CAD build for the part. Positions are in the model's coordinates, mm. A direction names the side the tool comes from. Give positions to 0.01 mm unless a question says otherwise; leave off trailing zeros. Write each loop counter-clockwise with the first axis right and the second up, starting at its lowest first coordinate (ties: lowest second). Pieces come first, ordered by that corner, then holes. Notation, with made-up numbers: (-34, -38.5) - (-16, -38.5) arc R21 ccw to (-16, -13.5) - close; hole circle Ø8 at (35, 54). An arc over 180 degrees is marked (long way). Answer as a JSON object with one key per item and string values.
from build123d import *

# Parameters (mm, degrees)
F0_R      = 13.1
F1_DEPTH  = 80
F2_R      = 9.5
F3_DEPTH  = 50
F4_R      = 6.6526235809
F5_DEPTH  = 25
F7_DEPTH  = 25
F8_R      = 0.75
F9_DEPTH  = 5
F10_W     = 4.01619326
F10_H     = 1.2
F11_DEPTH = 1
F13_DEPTH = 44
F14_DEPTH = 44
F15_DEPTH = 10
F16_DEPTH = 10


with BuildPart() as f1:
    # F0 (on Top) → F1 (new body)
    with BuildSketch(Plane.XY):
        Circle(F0_R)
    extrude(amount=F1_DEPTH)

    # F2 (on face) → F3 (cut)
    with BuildSketch(Plane.XY.offset(80)):
        Circle(F2_R)
    extrude(amount=-F3_DEPTH, mode=Mode.SUBTRACT)

    # F4 (on face) → F5 (cut)
    with BuildSketch(Plane.XY.offset(30)):
        Circle(F4_R)
    extrude(amount=-F5_DEPTH, mode=Mode.SUBTRACT)

    # F6 (on face) → F7 (join)
    with BuildSketch(Plane.XY.offset(5)):
        with BuildLine():
            ThreePointArc((2.00809663, 6.3423141229), (0, 6.6526235809), (-2.00809663, 6.3423141229))
            Line((-2.00809663, 6.3423141229), (-2.00809663, -6.3423141229))
            ThreePointArc((-2.00809663, -6.3423141229), (0, -6.6526235809), (2.00809663, -6.3423141229))
            Line((2.00809663, -6.3423141229), (2.00809663, 6.3423141229))
        make_face()
    extrude(amount=F7_DEPTH)

    # F8 (on face) → F9 (cut)
    with BuildSketch(Plane.XY.offset(5)):
        with Locations((-3.75, 0)):
            Circle(F8_R)
        with Locations((3.75, 0)):
            Circle(F8_R)
    extrude(amount=-F9_DEPTH, mode=Mode.SUBTRACT)

    # F10 (on face) → F11 (cut)
    with BuildSketch(Plane.XY.offset(30)):
        Rectangle(F10_W, F10_H)
    extrude(amount=-F11_DEPTH, mode=Mode.SUBTRACT)

    # F12 (on face) → F13 (cut)
    with BuildSketch(Plane.XY.offset(80)):
        with BuildLine():
            Line((-7.3388648552, 10.8513161708), (-4.4335485277, 8.4020025859))
            ThreePointArc((-4.4335485277, 8.4020025859), (1.034452264, 9.4435114504), (6.1473147231, 7.2429635989))
            Line((6.1473147231, 7.2429635989), (7.3388648552, 10.8513161708))
            ThreePointArc((7.3388648552, 10.8513161708), (0, 13.1), (-7.3388648552, 10.8513161708))
        make_face()
    extrude(amount=-F13_DEPTH, mode=Mode.SUBTRACT)

    # F12 (on face) → F14 (cut)
    with BuildSketch(Plane.XY.offset(80)):
        with BuildLine():
            ThreePointArc((4.4335485277, -8.4020025859), (-1.034452264, -9.4435114504), (-6.1473147231, -7.2429635989))
            Line((-6.1473147231, -7.2429635989), (-7.3388648552, -10.8513161708))
            ThreePointArc((-7.3388648552, -10.8513161708), (0, -13.1), (7.3388648552, -10.8513161708))
            Line((7.3388648552, -10.8513161708), (4.4335485277, -8.4020025859))
        make_face()
    extrude(amount=-F14_DEPTH, mode=Mode.SUBTRACT)

    # F12 (on face) → F15 (join)
    with BuildSketch(Plane.XY.offset(80)):
        with BuildLine():
            ThreePointArc((4.4335485277, -8.4020025859), (-1.034452264, -9.4435114504), (-6.1473147231, -7.2429635989))
            Line((-6.1473147231, -7.2429635989), (-7.3388648552, -10.8513161708))
            ThreePointArc((-7.3388648552, -10.8513161708), (0, -13.1), (7.3388648552, -10.8513161708))
            Line((7.3388648552, -10.8513161708), (4.4335485277, -8.4020025859))
        make_face()
    extrude(amount=-F15_DEPTH)

    # F12 (on face) → F16 (join)
    with BuildSketch(Plane.XY.offset(80)):
        with BuildLine():
            Line((-7.3388648552, 10.8513161708), (-4.4335485277, 8.4020025859))
            ThreePointArc((-4.4335485277, 8.4020025859), (1.034452264, 9.4435114504), (6.1473147231, 7.2429635989))
            Line((6.1473147231, 7.2429635989), (7.3388648552, 10.8513161708))
            ThreePointArc((7.3388648552, 10.8513161708), (0, 13.1), (-7.3388648552, 10.8513161708))
        make_face()
    extrude(amount=-F16_DEPTH)


solid = f1.part
(1) Probe L1, parallel to Z at x = -1, y = -9.75; L2, parallel to X at y = 1.5, z = 22; L3, parallel to X at y = 0, z = 53. List the from-to ranges inside material, lowest first. Write a range as [from, to].
Answer key:
{"L1": "z = [0, 36], [70, 80]", "L2": "x = [-13.01, -6.48], [-2.01, 2.01], [6.48, 13.01]", "L3": "x = [-13.1, -9.5], [9.5, 13.1]"}
(2) Pull direction Y, two halves, no side cores. Call faces 5 (the face through (3, 0, 3)), 6 (the face through (9, 4, 80)), 7 (the face through (-6.735, -9.022, 53.238)): pulls with the +Y half, pulls with the -Y half, needs draft (parallel to the pull), parting line crosses it, or undercut.
Answer key:
{"face 5": "undercut", "face 6": "needs draft", "face 7": "pulls with the -Y half"}
(3) Saw through at D-D, the plane x = -8.75. Give the cut face in (y, z).
Answer key:
{"outline": "(-9.75, 0) - (9.75, 0) - (9.75, 80) - (3.7, 80) - (3.7, 30) - (-3.7, 30) - (-3.7, 80) - (-9.75, 80) - close"}
(4) Saw through at B-B, the plane x = 0. Give the cut face in (y, z), and give its area (3 significant figures).
Answer key:
{"outline": "(-13.1, 0) - (13.1, 0) - (13.1, 36) - (9.5, 36) - (9.5, 30) - (0.6, 30) - (0.6, 29) - (-0.6, 29) - (-0.6, 30) - (-9.5, 30) - (-9.5, 36) - (-13.1, 36) - close; (-13.1, 70) - (-9.5, 70) - (-9.5, 80) - (-13.1, 80) - close; (9.5, 70) - (13.1, 70) - (13.1, 80) - (9.5, 80) - close", "area": "900 mm²"}
(5) Saw through at A-A, the plane z = 62. Give the cut face in (x, y), and give its area (3 significant figures).
Answer key:
{"outline": "(-7.34, -10.85) - (-6.15, -7.24) arc R9.5 cw to (-4.43, 8.4) - (-7.34, 10.85) arc R13.1 ccw to start; (4.43, -8.4) - (7.34, -10.85) arc R13.1 ccw to (7.34, 10.85) - (6.15, 7.24) arc R9.5 cw to start", "area": "159 mm²"}
(6) Saw through at C-C, the plane z = 21.5. Give the cut face in (x, y).
Answer key:
{"outline": "circle Ø26.2 at (0, 0); hole (-2.01, -6.34) - (-2.01, 6.34) arc R6.65 ccw to start; hole (2.01, -6.34) arc R6.65 ccw to (2.01, 6.34) - close"}
(7) 3-axis set-ups, long thin cutter, end or side, ignore diameter. For faces 1 (the face through (-5.907, 9.644, 53.238)), 2 (the face through (0, 0, 0)), 3 (the face through (0, -11, 70)), 4 (the face through (-5, 0, 5)): which of +Z, -Z, +X, -X, +Y, -Y reach the whole face in a straight line?
Answer key:
{"face 1": "+Y", "face 2": "-Z, +X, -X, +Y, -Y", "face 3": "-Y", "face 4": "+Z"}
(8) Flat gauge pins, fed straight in: P1, Ø2.5, axis at x = 4, y = 1.5, coming from the +Z side; P2, Ø1.5, axis at y = 10, z = 70, coming from the -X side; P3, Ø1.4, axis at x = 3.75, y = 0, coming from the +Z side; P4, Ø6.5, axis at x = 2.5, y = 9, coming from the +Z side. Where does each tip first touch, or does it go through?
Answer key:
{"P1": "stops at z = 5", "P2": "stops at x = -9.28", "P3": "passes through", "P4": "stops at z = 80"}
